Geometry check sheet. Reference: the model listing, model coordinates, mm. A direction names the side the tool comes from. Coordinates: 2 decimals unless noted, no trailing zeros. Loops run counter-clockwise (first coordinate to the right, second up) from the corner with the lowest first, then second, coordinate; pieces in that order, holes last.
from build123d import *

# Parameters (mm, degrees)
BOSS_EXTRU_2_DEPTH = 55
CONG_2_R           = 2


with BuildPart() as part:
    # Esquisse1 → Boss.-Extru.2 (new body)
    with BuildSketch(Plane.XY):
        with BuildLine():
            Line((33.25, 68), (33.25, 34))
            Line((33.25, 34), (33.25, 0))
            Line((33.25, 0), (0, 0))
            Line((0, 0), (0, -0.4))
            Line((0, -0.4), (33.65, -0.4))
            Line((33.65, -0.4), (33.65, 34))
            Line((33.65, 34), (33.65, 68))
            ThreePointArc((33.65, 68), (28.572164781, 71.359134798), (27.46710324, 65.37189536))
            Line((27.46710324, 65.37189536), (27.75, 65.65479212))
            ThreePointArc((27.75, 65.65479212), (28.725245122, 70.989565186), (33.25, 68))
        make_face()
    extrude(amount=BOSS_EXTRU_2_DEPTH)

    # Congé2
    cong_2_edges = [part.edges().sort_by_distance(p)[0] for p in [
        (33.25, 0, 27.5),
        (33.65, -0.4, 27.5),
    ]]
    fillet(cong_2_edges, radius=CONG_2_R)

    # Symétrie2: part across plane


with BuildPart() as part_1:
    add(part.part)
    add(part.part.mirror(Plane(origin=(0, -0.4, 55), x_dir=(0, 0, 1), z_dir=(1, 0, 0))))


solid = part_1.part
1) Section check A-A on x = 30. Record the cut outline in (y, z).
Data:
outline: (-0.4, 0) - (0, 0) - (0, 55) - (-0.4, 55) - close; (71.25, 0) - (71.65, 0) - (71.65, 55) - (71.25, 55) - close
2) Section check B-B on y = 8. Record the cut outline in (x, z), and give its area (3 significant figures).
Data:
outline: (-33.65, 0) - (-33.25, 0) - (-33.25, 55) - (-33.65, 55) - close; (33.25, 0) - (33.65, 0) - (33.65, 55) - (33.25, 55) - close
area: 44.0 mm2
3) Mould release check, pull along Y, two halves, no side actions. Record for faces 3 (the cylindrical face through (33.05, 0.17, 27.88)), 4 (the flat face through (-33.65, 34, 27)), 5 (the cylindrical face through (-28.64, 70.95, 27.12)): +Y half, -Y half, draft (parallel to the pull), parting line (faces both ways), or undercut.
Data:
face 3: -Y half
face 4: draft
face 5: undercut
4) Access from +Z, -Z, +X, -X, +Y, -Y to the whole of each face (thin tool, end or side, straight path). Record for faces 1 (the cylindrical face through (-33.05, 0.17, 27.88)), 2 (the cylindrical face through (-32.68, 0.6, 27.88)).
Data:
face 1: +Z, -Z, -X, -Y
face 2: +Z, -Z
5) Section check C-C on z = 48.5. Record the cut outline in (x, y), and give its area (3 significant figures).
Data:
outline: (-33.65, 1.6) arc R2 ccw to (-31.65, -0.4) - (31.65, -0.4) arc R2 ccw to (33.65, 1.6) - (33.65, 68) arc R3.65 ccw (long way) to (27.47, 65.37) - (27.75, 65.65) arc R3.25 cw (long way) to (33.25, 68) - (33.25, 2) arc R2 cw to (31.25, 0) - (-31.25, 0) arc R2 cw to (-33.25, 2) - (-33.25, 68) arc R3.25 cw (long way) to (-27.75, 65.65) - (-27.47, 65.37) arc R3.65 ccw (long way) to (-33.65, 68) - close
area: 92.2 mm2
6) Depth check by flat-ended pin: pin 1 (5 mm diameter, centred on x = -22.5, z = 23.5, fed in from +Y). Enter the tip coordinate at first touch or a pass-through.
Data:
pin 1: stops at y = 0
7) Section check D-D on x = -8. Record the cut outline in (y, z).
Data:
outline: (-0.4, 0) - (0, 0) - (0, 55) - (-0.4, 55) - close
8) Material ranges on probe 1 along X at (y, z) = (68, 43); probe 2 along X at (y, z) = (22.5, 11); probe 3 along Y at (x, z) = (-30, 13), recorded low to high.
Data:
probe 1: x = -33.65 to -33.25, -26.75 to -26.35, 26.35 to 26.75, 33.25 to 33.65
probe 2: x = -33.65 to -33.25, 33.25 to 33.65
probe 3: y = -0.4 to 0, 71.25 to 71.65
